Here's how the part is built. I have some questions about the finished solid (model axes, mm). A direction names the side the tool comes from. Round coordinates to 2 decimals unless told otherwise and drop trailing zeros. Order: outer loops, then holes, each group sorted by start corner. A loop starts at its lowest first (then second) coordinate and runs counter-clockwise, first axis right, second up. Notation, with made-up numbers: M -5.75,7.5 L 9.25,7.5 A26 cw 9.25,43.5 Z; hole C 28.25,7 d11. An arc over 180 degrees is marked long. Use one line per item in the form item = value. Start each with the question number.
```python
from build123d import *

# Parameters (mm, degrees)
F0_W     = 57.15
F0_H     = 44.45
F1_DEPTH = 25.4
F2_W     = 44.45
F2_H     = 31.75
F3_DEPTH = 25.4
F5_DEPTH = 25.4
F7_DEPTH = 25.4


with BuildPart() as f1:
    # F0 (on Front) → F1 (new body)
    with BuildSketch(Plane.XZ):
        with Locations((28.575, 22.225)):
            Rectangle(F0_W, F0_H)
    extrude(amount=F1_DEPTH)

    # F2 (on face) → F3 (cut)
    with BuildSketch(Plane.XZ.offset(25.4)):
        with Locations((34.925, 28.575)):
            Rectangle(F2_W, F2_H)
    extrude(amount=-F3_DEPTH, mode=Mode.SUBTRACT)

    # F4 (on face) → F5 (cut)
    with BuildSketch(Plane.YZ.offset(12.7)):
        with BuildLine():
            ThreePointArc((-19.05, 42.9509683429), (-15.9622689922, 44.0701615546), (-12.7, 44.45))
            Line((-12.7, 44.45), (-25.4, 44.45))
            Line((-25.4, 44.45), (-25.4, 36.6009683429))
            ThreePointArc((-25.4, 36.6009683429), (-22.740231571, 40.2911999139), (-19.05, 42.9509683429))
        make_face()
        with BuildLine():
            Line((0, 44.45), (-12.7, 44.45))
            ThreePointArc((-12.7, 44.45), (-9.4377310078, 44.0701615546), (-6.35, 42.9509683429))
            ThreePointArc((-6.35, 42.9509683429), (-2.659768429, 40.2911999139), (0, 36.6009683429))
            Line((0, 36.6009683429), (0, 44.45))
        make_face()
        with BuildLine():
            Line((-12.7, 36.6009683429), (-12.7, 44.45))
            ThreePointArc((-12.7, 44.45), (-15.9622689922, 44.0701615546), (-19.05, 42.9509683429))
            Line((-19.05, 42.9509683429), (-19.05, 30.2509683429))
            ThreePointArc((-19.05, 30.2509683429), (-17.1901280605, 34.7410964034), (-12.7, 36.6009683429))
        make_face()
        with BuildLine():
            ThreePointArc((-6.35, 42.9509683429), (-9.4377310078, 44.0701615546), (-12.7, 44.45))
            Line((-12.7, 44.45), (-12.7, 36.6009683429))
            ThreePointArc((-12.7, 36.6009683429), (-8.2098719395, 34.7410964034), (-6.35, 30.2509683429))
            Line((-6.35, 30.2509683429), (-6.35, 42.9509683429))
        make_face()
        with BuildLine():
            Line((-12.7, 23.9009683429), (-12.7, 30.2509683429))
            Line((-12.7, 30.2509683429), (-19.05, 30.2509683429))
            ThreePointArc((-19.05, 30.2509683429), (-17.1901280605, 25.7608402823), (-12.7, 23.9009683429))
        make_face()
        with BuildLine():
            Line((-12.7, 30.2509683429), (-12.7, 36.6009683429))
            ThreePointArc((-12.7, 36.6009683429), (-17.1901280605, 34.7410964034), (-19.05, 30.2509683429))
            Line((-19.05, 30.2509683429), (-12.7, 30.2509683429))
        make_face()
        with BuildLine():
            Line((-6.35, 30.2509683429), (-12.7, 30.2509683429))
            Line((-12.7, 30.2509683429), (-12.7, 23.9009683429))
            ThreePointArc((-12.7, 23.9009683429), (-8.2098719395, 25.7608402823), (-6.35, 30.2509683429))
        make_face()
        with BuildLine():
            ThreePointArc((-6.35, 30.2509683429), (-8.2098719395, 34.7410964034), (-12.7, 36.6009683429))
            Line((-12.7, 36.6009683429), (-12.7, 30.2509683429))
            Line((-12.7, 30.2509683429), (-6.35, 30.2509683429))
        make_face()
    extrude(amount=-F5_DEPTH, mode=Mode.SUBTRACT)

    # F6 (on face) → F7 (cut)
    with BuildSketch(Plane.XY.offset(12.7)):
        with BuildLine():
            ThreePointArc((31.6799919585, -11.7596803731), (29.5443618549, -7.8888915191), (25.4, -6.35))
            Line((25.4, -6.35), (25.4, -12.7))
            Line((25.4, -12.7), (31.6454185395, -12.7))
            ThreePointArc((31.6454185395, -12.7), (31.6540648134, -12.2295224974), (31.6799919585, -11.7596803731))
        make_face()
        with BuildLine():
            Line((25.4, -12.7), (25.4, -6.35))
            ThreePointArc((25.4, -6.35), (20.9098719395, -8.2098719395), (19.05, -12.7))
            Line((19.05, -12.7), (25.4, -12.7))
        make_face()
        with BuildLine():
            ThreePointArc((46.0831890214, 0), (44.45, 0.1045814605), (42.8168109786, 0))
            Line((42.8168109786, 0), (44.45, 0))
            Line((44.45, 0), (46.0831890214, 0))
        make_face()
        with BuildLine():
            Line((31.6454185395, -12.7), (25.4, -12.7))
            Line((25.4, -12.7), (25.4, -19.05))
            ThreePointArc((25.4, -19.05), (29.5443618549, -17.5111084809), (31.6799919585, -13.6403196269))
            ThreePointArc((31.6799919585, -13.6403196269), (31.6540648134, -13.1704775026), (31.6454185395, -12.7))
        make_face()
        with BuildLine():
            Line((25.4, -19.05), (25.4, -12.7))
            Line((25.4, -12.7), (19.05, -12.7))
            ThreePointArc((19.05, -12.7), (20.9098719395, -17.1901280605), (25.4, -19.05))
        make_face()
        with BuildLine():
            Line((57.15, 0), (46.0831890214, 0))
            ThreePointArc((46.0831890214, 0), (53.504206381, -3.645793619), (57.15, -11.0668109786))
            Line((57.15, -11.0668109786), (57.15, 0))
        make_face()
        with BuildLine():
            ThreePointArc((50.8, -12.7), (48.9401280605, -8.2098719395), (44.45, -6.35))
            Line((44.45, -6.35), (44.45, -12.7))
            Line((44.45, -12.7), (50.8, -12.7))
        make_face()
        with BuildLine():
            Line((44.45, -12.7), (44.45, -6.35))
            ThreePointArc((44.45, -6.35), (39.9598719395, -8.2098719395), (38.1, -12.7))
            Line((38.1, -12.7), (44.45, -12.7))
        make_face()
        with BuildLine():
            Line((44.45, -12.7), (38.1, -12.7))
            ThreePointArc((38.1, -12.7), (39.9598719395, -17.1901280605), (44.45, -19.05))
            Line((44.45, -19.05), (44.45, -12.7))
        make_face()
        with BuildLine():
            Line((50.8, -12.7), (44.45, -12.7))
            Line((44.45, -12.7), (44.45, -19.05))
            ThreePointArc((44.45, -19.05), (48.9401280605, -17.1901280605), (50.8, -12.7))
        make_face()
        with BuildLine():
            Line((57.15, -25.4), (57.15, -14.3331890214))
            ThreePointArc((57.15, -14.3331890214), (53.504206381, -21.754206381), (46.0831890214, -25.4))
            Line((46.0831890214, -25.4), (57.15, -25.4))
        make_face()
    extrude(amount=-F7_DEPTH, mode=Mode.SUBTRACT)


solid = f1.part
```
1) If we section it at C-C on z = 5.5: Write out the boundary of the cut face in (x, y).
2) If I drill on line 1 (Y direction, x = 25.5, z = 4.5); line 2 (Z direction, x = 34.5, y = -18.25), over which ranges is the centre line in solid material (lowest first)?
3) On a 3-axis mill with a long thin cutter (end or side, diameter ignored), from which of +Z, -Z, +X, -X, +Y, -Y can I reach the whole of each face in a straight line? I mean faces 5 (the flat face through (35, -13, 12.7)), 6 (the flat face through (57.15, -13, 6)). Say none if no direction works.
4) If we section it at A-A on y = -10: Write out the boundary of the cut face in (x, z).
5) Will these pins go through, and if not, where does the flat tip stop? pin 1 Ø12.5 at (x, y) = (30.5, -9.5) entering from +Z; pin 2 Ø8 at (y, z) = (-10.5, 28.5) entering from +X; pin 3 Ø1 at (x, z) = (47, 10) entering from +Y.
6) If we section it at B-B on z = 37.5: Write out the boundary of the cut face in (x, y).
7) If we section it at D-D on y = -17.25: Write out the boundary of the cut face in (x, z), then the cut area to 3 significant figures.
8) If we mould it in two halves opening along Y, with no side actions, what happens to faces 1 (the flat face through (6, -19.05, 37)), 2 (the cylindrical face through (53.42, -3.56, 6.44)), 3 (the flat face through (6, -6.35, 37)), 4 (the flat face through (22, -7, 0))? For each: +Y half, -Y half, draft (parallel to the pull), parting line (faces both ways), or undercut.
Completed:
q1.outline = M 0,-25.4 L 46.08,-25.4 A12.8 ccw 57.15,-14.33 L 57.15,-11.07 A12.8 ccw 46.08,0 L 0,0 Z; hole M 31.68,-13.64 A12.8 cw 31.68,-11.76 A6.35 ccw long Z; hole C 44.45,-12.7 d12.7
q2.line_1 = -25.4 to -19.05, -6.35 to 0
q2.line_2 = 0 to 12.7
q3.face_5 = +Z, +X, +Y, -Y
q3.face_6 = +Z, -Z, +X, +Y, -Y
q4.outline = M 0,0 L 19.65,0 L 19.65,12.7 L 12.7,12.7 L 12.7,24.5 L 0,24.5 Z; M 31.15,0 L 38.7,0 L 38.7,12.7 L 31.15,12.7 Z; M 50.2,0 L 56.97,0 L 56.97,12.7 L 50.2,12.7 Z
q5.pin_1 = 12.7
q5.pin_2 = 12.7
q5.pin_3 = -0.06
q6.outline = M 0,-24.91 L 12.7,-24.91 L 12.7,-19.05 L 0,-19.05 Z; M 0,-6.35 L 12.7,-6.35 L 12.7,-0.49 L 0,-0.49 Z
q7.outline = M 0,0 L 20.97,0 L 20.97,12.7 L 12.7,12.7 L 12.7,25.82 L 0,25.82 Z; M 29.83,0 L 40.02,0 L 40.02,12.7 L 29.83,12.7 Z; M 48.88,0 L 56.42,0 L 56.42,12.7 L 48.88,12.7 Z
q7.area = 658 mm²
q8.face_1 = undercut
q8.face_2 = +Y half
q8.face_3 = undercut
q8.face_4 = draft
